```python
from build123d import *

# Parameters (mm, degrees)
F1_DEPTH  = 1
F3_DEPTH  = 40
F5_DEPTH  = 7.6454254
F8_DEPTH  = 8.9916
F9_DEPTH  = 39.37
F11_REACH = 42.1217729552
F13_REACH = 63.4368099505
F15_REACH = 84.7531019793
F16_W     = 9.9314
F16_H     = 11.938
F17_DEPTH = 2
F18_W     = 9.9314
F18_H     = 11.938
F19_DEPTH = 2
F20_R     = 2
F22_D     = 4.5


with BuildPart() as f1:
    # F0 (on Top) → F1 (new body, symmetric)
    with BuildSketch(Plane.XY):
        Polygon((40, -50), (40, 50), (10.4203875556, 50), (10.4203875556, 63.4358227253), (0, 63.4358227253), (0, 50), (0, 40.4320432043), (20.8407751113, 40.4320432043), (20.8407751113, 19.8559855986), (0, 19.8559855986), (0, 10.2880288029), (20.8407751113, 10.2880288029), (20.8407751113, -10.2880288029), (0, -10.2880288029), (0, -19.8559855986), (20.8407751113, -19.8559855986), (20.8407751113, -40.4320432043), (0, -40.4320432043), (0, -50), align=None)
    extrude(amount=F1_DEPTH, both=True)

    # F2 (on Right) → F3 (join)
    with BuildSketch(Plane.YZ):
        Polygon((-50, 1), (-50, 0.9964082731), (-44.6311706177, 6.3652376554), (-46.04538418, 7.7794512178), (-51.4515079706, 2.3733274272), align=None)
    extrude(amount=-F3_DEPTH)

    # F4 (on face) → F5 (join)
    with BuildSketch(Plane(origin=(0, -19.1329664811, -19.1329664811), x_dir=(1, 0, 0), z_dir=(0, 0.7071067812, 0.7071067812))):
        with BuildLine():
            Line((-34.9300994608, -32.0862576741), (-40.6840402867, -34.1805208645))
            ThreePointArc((-40.6840402867, -34.1805208645), (-41.969615506, -36.4072024614), (-40, -38.059906106))
            Line((-40, -38.059906106), (-40, -36.059906106))
            Line((-40, -36.059906106), (-34.2460591741, -33.9656429157))
            Line((-34.2460591741, -33.9656429157), (-34.9300994608, -32.0862576741))
        make_face()
    extrude(amount=-F5_DEPTH)

    # F6 (on Right) + F2 (on Right) + F7 (on Right) → F8 (join)
    with BuildSketch(Plane.YZ):
        Polygon((-19.8559855986, 0.9982251152), (-19.8559855986, 0.9946333883), (-14.4871562162, 6.3634627706), (-15.9013697786, 7.777676333), (-21.3074935692, 2.3715525424), align=None)
        with BuildLine():
            Line((-19.8559855986, -1), (-19.8559855986, 0.9946333883))
            Line((-19.8559855986, 0.9946333883), (-19.8559855986, 0.9982251152))
            Line((-19.8559855986, 0.9982251152), (-21.3074935692, 2.3715525424))
            ThreePointArc((-21.3074935692, 2.3715525424), (-21.6913494545, 0.2080712521), (-19.8559855986, -1))
        make_face()
    with BuildSketch(Plane.YZ):
        Polygon((-50, 1), (-50, 0.9964082731), (-44.6311706177, 6.3652376554), (-46.04538418, 7.7794512178), (-51.4515079706, 2.3733274272), align=None)
        with BuildLine():
            Line((-50, -0.9982251152), (-50, 0.9964082731))
            Line((-50, 0.9964082731), (-50, 1))
            Line((-50, 1), (-51.4515079706, 2.3733274272))
            ThreePointArc((-51.4515079706, 2.3733274272), (-51.8353638559, 0.2098461369), (-50, -0.9982251152))
        make_face()
    with BuildSketch(Plane.YZ):
        Polygon((10.2880288029, 0.9982251152), (10.2880288029, 0.9946333883), (15.6568581852, 6.3634627706), (14.2426446228, 7.777676333), (8.8365208322, 2.3715525424), align=None)
        with BuildLine():
            Line((10.2880288029, -1), (10.2880288029, 0.9946333883))
            Line((10.2880288029, 0.9946333883), (10.2880288029, 0.9982251152))
            Line((10.2880288029, 0.9982251152), (8.8365208322, 2.3715525424))
            ThreePointArc((8.8365208322, 2.3715525424), (8.4526649469, 0.2080712521), (10.2880288029, -1))
        make_face()
        Polygon((40.4320432043, 1), (40.4320432043, 0.9964082731), (45.8008725867, 6.3652376554), (44.3866590243, 7.7794512177), (38.9805352337, 2.3733274272), align=None)
        with BuildLine():
            Line((40.4320432043, -0.9982251152), (40.4320432043, 0.9964082731))
            Line((40.4320432043, 0.9964082731), (40.4320432043, 1))
            Line((40.4320432043, 1), (38.9805352337, 2.3733274272))
            ThreePointArc((38.9805352337, 2.3733274272), (38.5966793484, 0.2098461369), (40.4320432043, -0.9982251152))
        make_face()
    extrude(amount=F8_DEPTH)

    # F6 (on Right) + F7 (on Right) → F9 (join)
    with BuildSketch(Plane.YZ):
        Polygon((-19.8559855986, 0.9982251152), (-19.8559855986, 0.9946333883), (-14.4871562162, 6.3634627706), (-15.9013697786, 7.777676333), (-21.3074935692, 2.3715525424), align=None)
    with BuildSketch(Plane.YZ):
        Polygon((10.2880288029, 0.9982251152), (10.2880288029, 0.9946333883), (15.6568581852, 6.3634627706), (14.2426446228, 7.777676333), (8.8365208322, 2.3715525424), align=None)
        Polygon((40.4320432043, 1), (40.4320432043, 0.9964082731), (45.8008725867, 6.3652376554), (44.3866590243, 7.7794512177), (38.9805352337, 2.3733274272), align=None)
    extrude(amount=-F9_DEPTH)

    f11_end = Plane(origin=(-19.685, -20.5817395839, 1.6848888288), x_dir=(0, -0.7263986223, 0.6872736293), z_dir=(0, -0.6872736293, -0.7263986223))
    # F10 (on face) → F11 (join, up to a plane its end follows)
    with BuildSketch(Plane(origin=(0, -4.0618467228, -4.0618467228), x_dir=(-1, 0, 0), z_dir=(0, 0.7071067812, 0.7071067812))):
        with BuildLine():
            Line((34.3000994608, 10.7699656456), (40.0540402867, 12.8642288359))
            ThreePointArc((40.0540402867, 12.8642288359), (41.339615506, 15.0909104328), (39.37, 16.7436140775))
            Line((39.37, 16.7436140775), (39.37, 14.7436140775))
            Line((39.37, 14.7436140775), (33.6160591741, 12.6493508872))
            Line((33.6160591741, 12.6493508872), (34.3000994608, 10.7699656456))
        make_face()
    f11_long = extrude(amount=-F11_REACH, mode=Mode.PRIVATE)
    add(split(f11_long, bisect_by=f11_end, keep=Keep.BOTTOM, mode=Mode.PRIVATE))

    f13_end = Plane(origin=(-19.685, 9.5622748176, 1.6848888288), x_dir=(0, -0.7263986223, 0.6872736293), z_dir=(0, -0.6872736293, -0.7263986223))
    # F12 (on face) → F13 (join, up to a plane its end follows)
    with BuildSketch(Plane(origin=(0, 11.0101604779, 11.0101604779), x_dir=(1, 0, 0), z_dir=(0, 0.7071067812, 0.7071067812))):
        with BuildLine():
            Line((-34.3000994608, 10.5450713499), (-40.0540402867, 8.4508081595))
            ThreePointArc((-40.0540402867, 8.4508081595), (-41.339615506, 6.2241265626), (-39.37, 4.5714229179))
            Line((-39.37, 4.5714229179), (-39.37, 6.5714229179))
            Line((-39.37, 6.5714229179), (-33.6160591741, 8.6656861083))
            Line((-33.6160591741, 8.6656861083), (-34.3000994608, 10.5450713499))
        make_face()
    f13_long = extrude(amount=-F13_REACH, mode=Mode.PRIVATE)
    add(split(f13_long, bisect_by=f13_end, keep=Keep.BOTTOM, mode=Mode.PRIVATE))

    f15_end = Plane(origin=(-19.685, 39.706289219, 1.6866637136), x_dir=(0, -0.7263986223, 0.6872736293), z_dir=(0, -0.6872736293, -0.7263986223))
    # F14 (on face) → F15 (join, up to a plane its end follows)
    with BuildSketch(Plane(origin=(0, 26.0830551211, 26.083055121), x_dir=(-1, 0, 0), z_dir=(0, 0.7071067812, 0.7071067812))):
        with BuildLine():
            Line((34.3000994608, -31.8588533121), (40.0540402867, -29.7645901218))
            ThreePointArc((40.0540402867, -29.7645901218), (41.339615506, -27.5379085249), (39.37, -25.8852048802))
            Line((39.37, -25.8852048802), (39.37, -27.8852048802))
            Line((39.37, -27.8852048802), (33.6160591741, -29.9794680706))
            Line((33.6160591741, -29.9794680706), (34.3000994608, -31.8588533121))
        make_face()
    f15_long = extrude(amount=-F15_REACH, mode=Mode.PRIVATE)
    add(split(f15_long, bisect_by=f15_end, keep=Keep.BOTTOM, mode=Mode.PRIVATE))

    # F16 (on face) → F17 (join)
    with BuildSketch(Plane(origin=(0, 50, 0), x_dir=(-1, 0, 0), z_dir=(0, 1, 0))):
        with Locations((-28.5319, 4.969)):
            Rectangle(F16_W, F16_H)
    extrude(amount=F17_DEPTH)

    # F18 (on face) → F19 (join)
    with BuildSketch(Plane.XZ.offset(50)):
        with Locations((28.5319, 4.969)):
            Rectangle(F18_W, F18_H)
    extrude(amount=F19_DEPTH)

    # F20
    f20_edges = [f1.edges().sort_by_distance(p)[0] for p in [
        (28.5319, -52, -1),
        (28.5319, 52, -1),
    ]]
    fillet(f20_edges, radius=F20_R)

    # F22 (through all)
    with Locations(Plane.XZ.offset(52)):
        with Locations((28.5319, 5.9723)):
            Hole(F22_D / 2)


solid = f1.part
```
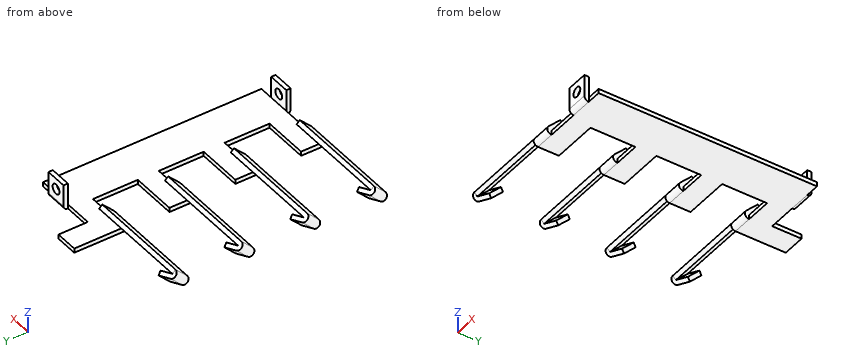
Could you check a few things on this model? Use its own coordinates, in mm. Round coordinates to 2 decimals unless told otherwise and drop trailing zeros. Loops run counter-clockwise (first coordinate to the right, second up) from the corner with the lowest first, then second, coordinate; pieces in that order, holes last. Notation, with made-up numbers: M 7,24 L 61,24 A18 ccw 61,28 Z; hole C 38,61.25 d5. An arc over 180 degrees is marked long. Write item = value, one per line.
1. I want a section at A-A, the plane x = -22.5. Count the separate pieces of the cut face and the enclosed holes in it, and give its area (3 significant figures).
Results below:
separate_pieces = 4
enclosed_holes = 0
area = 60.9 mm²
2. I want a section at C-C, the plane y = 7. Write out the boundary of the cut face in (x, z).
Results below:
outline = M 20.84,-1 L 40,-1 L 40,1 L 20.84,1 Z
3. I want a section at B-B, the plane x = 15.5. Write out the boundary of the cut face in (y, z).
Results below:
outline = M -50,-1 L -40.43,-1 L -40.43,1 L -50,1 Z; M -19.86,-1 L -10.29,-1 L -10.29,1 L -19.86,1 Z; M 10.29,-1 L 19.86,-1 L 19.86,1 L 10.29,1 Z; M 40.43,-1 L 50,-1 L 50,1 L 40.43,1 Z
4. Will these pins go through, and if not, where does the flat tip stop? P1, Ø2, axis at y = 42, z = 4, coming from the +X side; P2, Ø6, axis at x = -20, y = -14.5, coming from the +Z side; P3, Ø1.6, axis at y = -26, z = 0, coming from the -X side.
Results below:
P1 = 8.99
P2 = 7.78
P3 = 20.84
5. I need wall thicknesses on probe 1 along Y at (x, z) = (-7, 5.5); probe 2 along Y at (x, z) = (3.5, 2.25); probe 3 along Y at (x, z) = (26, 10). Which ranges of each line are inside material? Lowest first, please.
Results below:
probe_1 = -48.32 to -45.5, -18.18 to -15.35, 11.96 to 14.79, 42.11 to 44.94
probe_2 = -51.56 to -48.75, -21.41 to -18.6, 8.73 to 11.54, 38.87 to 41.69
probe_3 = -52 to -50, 50 to 52
